Work out the finished part from the listing and answer in its coordinate system (mm). Face numbers are marked on the shaded views. A direction names the side the tool comes from. Give positions to 0.01 mm unless a question says otherwise; leave off trailing zeros. Order: outer loops, then holes, each group sorted by start corner. A loop starts at its lowest first (then second) coordinate and runs counter-clockwise, first axis right, second up.
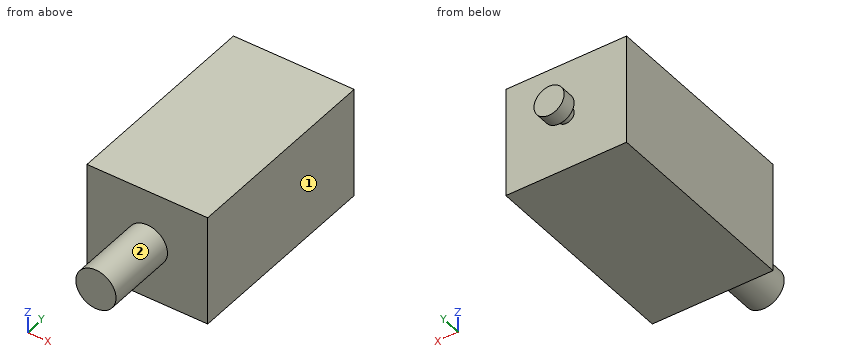
```python
from build123d import *

# Parameters (mm, degrees)
F0_W     = 12
F0_H     = 11
F1_DEPTH = 20.5
F2_R     = 2
F3_DEPTH = 7.2
F4_R     = 0.8
F5_DEPTH = 1
F6_R     = 1.5
F6_R_2   = 0.8
F7_DEPTH = 1.4


with BuildPart() as f1:
    # F0 (on Front) → F1 (new body)
    with BuildSketch(Plane.XZ):
        Rectangle(F0_W, F0_H)
    extrude(amount=F1_DEPTH)

    # F2 (on face) → F3 (join)
    with BuildSketch(Plane.XZ.offset(20.5)):
        Circle(F2_R)
    extrude(amount=F3_DEPTH)

    # F4 (on face) → F5 (join)
    with BuildSketch(Plane(origin=(0, 0, 0), x_dir=(-1, 0, 0), z_dir=(0, 1, 0))):
        Circle(F4_R)
    extrude(amount=F5_DEPTH)

    # F6 (on face) → F7 (join)
    with BuildSketch(Plane(origin=(0, 1, 0), x_dir=(-1, 0, 0), z_dir=(0, 1, 0))):
        Circle(F6_R)
        Circle(F6_R_2, mode=Mode.SUBTRACT)
        Circle(F6_R_2)
    extrude(amount=F7_DEPTH)


solid = f1.part
```
1. Which of the six approach directions +Z, -Z, +X, -X, +Y, -Y give full straight-line access (tool end or side, diameter ignored) to the marked faces 1 and 2?
Findings below:
face 1: +Z, -Z, +X, +Y, -Y
face 2: -Y
2. The part is cut by section A-A (x = 0). Write down the section's boundary in (y, z).
Findings below:
outline: (-27.7, -2) - (-20.5, -2) - (-20.5, -5.5) - (0, -5.5) - (0, -0.8) - (1, -0.8) - (1, -1.5) - (2.4, -1.5) - (2.4, 1.5) - (1, 1.5) - (1, 0.8) - (0, 0.8) - (0, 5.5) - (-20.5, 5.5) - (-20.5, 2) - (-27.7, 2) - close
3. The part is cut by section B-B (z = 0). Write down the section's boundary in (x, y), then the cut area to 3 significant figures.
Findings below:
outline: (-6, -20.5) - (-2, -20.5) - (-2, -27.7) - (2, -27.7) - (2, -20.5) - (6, -20.5) - (6, 0) - (0.8, 0) - (0.8, 1) - (1.5, 1) - (1.5, 2.4) - (-1.5, 2.4) - (-1.5, 1) - (-0.8, 1) - (-0.8, 0) - (-6, 0) - close
area: 281 mm2
4. Straight lines are drawn through the part: probe 1 along Y at (x, z) = (-4.5, -3); probe 2 along Z at (x, y) = (0, 0.5); probe 3 along Z at (x, y) = (-1.25, -26). For each, find the intervals that lie inside material, in ascending order.
Findings below:
probe 1: y = -20.5 to 0
probe 2: z = -0.8 to 0.8
probe 3: z = -1.56 to 1.56
5. Given P1, Ø3, axis at x = 3, z = -4.5, coming from the -Y side, flat-ended and moving along its own axis, determine where the tip first touches the part or whether it passes through.
Findings below:
P1: stops at y = -20.5
6. The part is cut by section C-C (x = -2.75). Write down the section's boundary in (y, z).
Findings below:
outline: (-20.5, -5.5) - (0, -5.5) - (0, 5.5) - (-20.5, 5.5) - close
7. The part is cut by section D-D (z = 3.75). Write down the section's boundary in (x, y), then the cut area to 3 significant figures.
Findings below:
outline: (-6, -20.5) - (6, -20.5) - (6, 0) - (-6, 0) - close
area: 246 mm2
